Input: part model. Units: mm. Frame: model coordinates. A direction names the side the tool comes from. Round coordinates to 2 decimals unless told otherwise and drop trailing zeros. Write each loop counter-clockwise with the first axis right and the second up, starting at its lowest first coordinate (ties: lowest second). Pieces come first, ordered by that corner, then holes. Notation, with made-up numbers: (28.5, -8) -> (80.5, -8) arc R25 ccw to (80.5, 24) -> close; hole circle Ø3 at (-37, -36). An arc over 180 degrees is marked (long way). Write item = value, one per line. Start each with the question number.
```python
from build123d import *

# Parameters (mm, degrees)
SKETCH_1_W               = 86
SKETCH_1_H               = 86
SKETCH_1_W_2             = 82
SKETCH_1_H_2             = 82
EXTRUDE_1_DEPTH          = 25
CUT_EXTRUDE_1_DEPTH      = 100.347873656
CUT_EXTRUDE_1_DEPTH_BACK = 28
SKETCH_2_R               = 3.75
FILLET_1_R               = 1
SKETCH_4_W               = 7.5
SKETCH_4_H               = 3.5
SKETCH_4_W_2             = 19
SKETCH_4_H_2             = 14.5
CUT_EXTRUDE_2_DEPTH      = 28
CHAMFER_1_SIZE           = 1
CHAMFER_2_SIZE           = 1
FILLET_2_R               = 2
SKETCH_9_W               = 6
SKETCH_9_H               = 15
EXTRUDE_2_DEPTH          = 6
SKETCH_13_W              = 6
SKETCH_13_H              = 15
EXTRUDE_3_DEPTH          = 6
SKETCH_14_W              = 6
SKETCH_14_H              = 15
EXTRUDE_4_DEPTH          = 6
SKETCH_15_R              = 2.5
CUT_EXTRUDE_5_DEPTH      = 12
FILLET_3_R               = 2
SKETCH_16_W              = 30
SKETCH_16_H              = 15
EXTRUDE_5_DEPTH          = 2
CHAMFER_3_SIZE           = 1
EXTRUDE_6_DEPTH          = 1.5
SKETCH_20_R              = 2.5
CUT_EXTRUDE_6_DEPTH      = 83.645326547


with BuildPart() as part:
    # Sketch 1 → Extrude 1 (new body)
    with BuildSketch(Plane(origin=(0, 0, 0), x_dir=(1, 0, 0), z_dir=(0, 1, 0))):
        Rectangle(SKETCH_1_W, SKETCH_1_H)
        Rectangle(SKETCH_1_W_2, SKETCH_1_H_2, mode=Mode.SUBTRACT)
    extrude(amount=EXTRUDE_1_DEPTH)

    # Sketch 2 → Cut-Extrude 1 (cut, two sides: drawn at the far end of the back side and taken through both)
    with BuildSketch(Plane.ZY.offset(43).offset(-CUT_EXTRUDE_1_DEPTH_BACK)):
        with Locations(Location((0, 12.5, 0), (0, 0, 180))):
            Circle(SKETCH_2_R)
        with Locations(Location((20, 12.5, 0), (0, 0, 180))):
            Circle(SKETCH_2_R)
        with Locations(Location((-20, 12.5, 0), (0, 0, 180))):
            Circle(SKETCH_2_R)
    extrude(amount=CUT_EXTRUDE_1_DEPTH + CUT_EXTRUDE_1_DEPTH_BACK, mode=Mode.SUBTRACT)

    # Fillet 1
    fillet_1_edges = [part.edges().sort_by_distance(p)[0] for p in [
        (-43, 12.5, -16.25),
        (-43, 12.5, 23.75),
        (-43, 12.5, 3.75),
    ]]
    fillet(fillet_1_edges, radius=FILLET_1_R)

    # Sketch 4 → Cut-Extrude 2 (cut)
    with BuildSketch(Plane(origin=(43, 0, 0), x_dir=(0, 0, -1), z_dir=(1, 0, 0))):
        with Locations((19.25, 13.25)):
            Rectangle(SKETCH_4_W, SKETCH_4_H)
        with Locations((-21.5, 12.5)):
            Rectangle(SKETCH_4_W_2, SKETCH_4_H_2)
    extrude(amount=-CUT_EXTRUDE_2_DEPTH, mode=Mode.SUBTRACT)

    # Chamfer 1
    chamfer_1_edges = [part.edges().sort_by_distance(p)[0] for p in [
        (43, 13.25, -15.5),
        (43, 11.5, -19.25),
        (43, 13.25, -23),
        (43, 15, -19.25),
    ]]
    chamfer(chamfer_1_edges, length=CHAMFER_1_SIZE)

    # Chamfer 2
    chamfer_2_edges = [part.edges().sort_by_distance(p)[0] for p in [
        (41, 19.75, 21.5),
        (41, 12.5, 31),
        (41, 5.25, 21.5),
        (41, 12.5, 12),
    ]]
    chamfer(chamfer_2_edges, length=CHAMFER_2_SIZE)

    # Fillet 2
    fillet_2_edges = [part.edges().sort_by_distance(p)[0] for p in [
        (43, 12.5, 43),
        (-43, 12.5, 43),
        (-43, 12.5, -43),
        (43, 12.5, -43),
    ]]
    fillet(fillet_2_edges, radius=FILLET_2_R)

    # Sketch 9 → Extrude 2 (add)
    with BuildSketch(Plane(origin=(-41, 0, 0), x_dir=(0, 0, -1), z_dir=(1, 0, 0))):
        with Locations((-38, 17.5)):
            Rectangle(SKETCH_9_W, SKETCH_9_H)
    extrude(amount=EXTRUDE_2_DEPTH)

    # Sketch 13 → Extrude 3 (add)
    with BuildSketch(Plane(origin=(-41, 0, 0), x_dir=(0, 0, -1), z_dir=(1, 0, 0))):
        with Locations((38, 17.5)):
            Rectangle(SKETCH_13_W, SKETCH_13_H)
    extrude(amount=EXTRUDE_3_DEPTH)

    # Sketch 14 → Extrude 4 (add)
    with BuildSketch(Plane.ZY.offset(-41)):
        with Locations((38, 17.5)):
            Rectangle(SKETCH_14_W, SKETCH_14_H)
        with Locations((-38, 17.5)):
            Rectangle(SKETCH_14_W, SKETCH_14_H)
    extrude(amount=EXTRUDE_4_DEPTH)

    # Sketch 15 → Cut-Extrude 5 (cut)
    with BuildSketch(Plane(origin=(0, 25, 0), x_dir=(1, 0, 0), z_dir=(0, 1, 0))):
        with Locations(Location((-39, 39, 0), (0, 0, 270))):
            Circle(SKETCH_15_R)
        with Locations(Location((39, 39, 0), (0, 0, 90))):
            Circle(SKETCH_15_R)
        with Locations(Location((39, -39, 0), (0, 0, 270))):
            Circle(SKETCH_15_R)
        with Locations(Location((-39, -39, 0), (0, 0, 90))):
            Circle(SKETCH_15_R)
    extrude(amount=-CUT_EXTRUDE_5_DEPTH, mode=Mode.SUBTRACT)

    # Fillet 3
    fillet_3_edges = [part.edges().sort_by_distance(p)[0] for p in [
        (-38, 10, 35),
        (-35, 10, 38),
        (-35, 17.5, 35),
        (-38, 10, -35),
        (-35, 17.5, -35),
        (-35, 10, -38),
        (38, 10, 35),
        (35, 17.5, 35),
        (35, 10, 38),
        (38, 10, -35),
        (35, 10, -38),
        (35, 17.5, -35),
    ]]
    fillet(fillet_3_edges, radius=FILLET_3_R)

    # Sketch 16 → Extrude 5 (add)
    with BuildSketch(Plane(origin=(0, 0, -43), x_dir=(-1, 0, 0), z_dir=(0, 0, -1))):
        with Locations((0, 12.5)):
            Rectangle(SKETCH_16_W, SKETCH_16_H)
    extrude(amount=EXTRUDE_5_DEPTH)

    # Chamfer 3
    chamfer_3_edges = [part.edges().sort_by_distance(p)[0] for p in [
        (-15, 12.5, -45),
        (0, 20, -45),
        (15, 12.5, -45),
        (0, 5, -45),
    ]]
    chamfer(chamfer_3_edges, length=CHAMFER_3_SIZE)

    # Sketch 19 → Extrude 6 (add, symmetric)
    with BuildSketch(Plane(origin=(0, 0, 0), x_dir=(0, 0, -1), z_dir=(1, 0, 0))):
        with BuildLine():
            Line((45, 17.5), (60, 17.5))
            ThreePointArc((60, 17.5), (65, 12.5), (60, 7.5))
            Line((60, 7.5), (45, 7.5))
            Line((45, 7.5), (45, 17.5))
        make_face()
    extrude(amount=EXTRUDE_6_DEPTH, both=True)

    # Sketch 20 → Cut-Extrude 6 (cut, through all)
    with BuildSketch(Plane.ZY.offset(1.5)):
        with Locations((-60, 12.5)):
            Circle(SKETCH_20_R)
    extrude(amount=-CUT_EXTRUDE_6_DEPTH, mode=Mode.SUBTRACT)


solid = part.part
```
1. Section A-A (x = 39). Output: boundary loops of the cut face in (y, z), then the cut area to 3 significant figures.
2. Section D-D (y = 2.25). Output: boundary loops of the cut face in (x, z), then the cut area to 3 significant figures.
3. Reachability of faces 1 (the flat face through (-39, 10, 39)), 2 (the flat face through (-35, 19, 39)), 3 (the flat face through (39, 13, 39)) from +Z, -Z, +X, -X, +Y, -Y: full face, straight path, thin tool, end or side. Return the list, or none.
4. Line query: line 1 along X through (y, z) = (16.75, 39); line 2 along Z through (x, y) = (-12, 17.5); line 3 along X through (y, z) = (22, -6.5). Output: solid intervals per line, ascending.
5. Section B-B (z = 0). Output: boundary loops of the cut face in (x, y).
6. Mould query, pull axis X, two halves, no side actions, for faces 4 (the flat face through (-1, 21, -43)), 5 (the flat face through (43, 12, 1)), 6 (the flat face through (-39, 10, -39)), 7 (the flat face through (41, 12, 1)). Classes: pulls with the +X half, pulls with the -X half, needs draft (parallel to the pull), parting line crosses it, or undercut.
7. Pin query (flat end, axial travel): P1, Ø12.5, axis at x = 3.5, y = 9.5, coming from the -Z side; P2, Ø5, axis at x = 15, y = 14.5, coming from the -Z side; P3, Ø3, axis at x = 24.5, y = 7.5, coming from the -Z side; P4, Ø12, axis at x = 12, z = -30, coming from the -Y side. Return the tip coordinate at first contact, or that it passes through.
8. Section C-C (z = 20). Output: boundary loops of the cut face in (x, y), then the cut area to 3 significant figures.
Check sheet entries:
q1.outline = (0, -43) -> (25, -43) -> (25, -41.5) -> (13, -41.5) -> (13, -36.5) -> (25, -36.5) -> (25, -35) -> (12, -35) arc R2 ccw to (10, -37) -> (10, -41) -> (0, -41) -> close; (0, 41) -> (10, 41) -> (10, 37) arc R2 ccw to (12, 35) -> (25, 35) -> (25, 36.5) -> (13, 36.5) -> (13, 41.5) -> (25, 41.5) -> (25, 43) -> (0, 43) -> close
q1.area = 158 mm2
q2.outline = (-43, -41) arc R2 ccw to (-41, -43) -> (41, -43) arc R2 ccw to (43, -41) -> (43, 41) arc R2 ccw to (41, 43) -> (-41, 43) arc R2 ccw to (-43, 41) -> close; hole (-41, -41) -> (41, -41) -> (41, 41) -> (-41, 41) -> close
q2.area = 669 mm2
q3.face_1 = -Y
q3.face_2 = +Y, -Y
q3.face_3 = +Y
q4.line_1 = -43 to -41.5, -36.5 to -35, 35 to 36.5, 41.5 to 43
q4.line_2 = -45 to -41, 41 to 43
q4.line_3 = -43 to -41, 41 to 43
q5.outline = (-43, 0) -> (-41, 0) -> (-41, 8.75) -> (-42, 8.75) arc R1 ccw to (-43, 7.75) -> close; (-43, 17.25) arc R1 ccw to (-42, 16.25) -> (-41, 16.25) -> (-41, 25) -> (-43, 25) -> close; (41, 0) -> (43, 0) -> (43, 25) -> (41, 25) -> close
q6.face_4 = needs draft
q6.face_5 = pulls with the +X half
q6.face_6 = undercut
q6.face_7 = undercut
q7.P1 = -65
q7.P2 = -45
q7.P3 = -43
q7.P4 = through
q8.outline = (-43, 0) -> (-41, 0) -> (-41, 8.75) -> (-42, 8.75) arc R1 ccw to (-43, 7.75) -> close; (-43, 17.25) arc R1 ccw to (-42, 16.25) -> (-41, 16.25) -> (-41, 25) -> (-43, 25) -> close; (41, 0) -> (43, 0) -> (43, 5.25) -> (42, 5.25) -> (41, 4.25) -> close; (41, 20.75) -> (42, 19.75) -> (43, 19.75) -> (43, 25) -> (41, 25) -> close
q8.area = 54.6 mm2
